Geometry: final body of the model. Coordinates: model frame, mm. Face numbers are marked on the shaded views. A direction names the side the tool comes from. Give positions to 0.01 mm unless a question says otherwise; leave off trailing zeros. Loops run counter-clockwise (first coordinate to the right, second up) from the corner with the lowest first, then second, coordinate; pieces in that order, holes last.
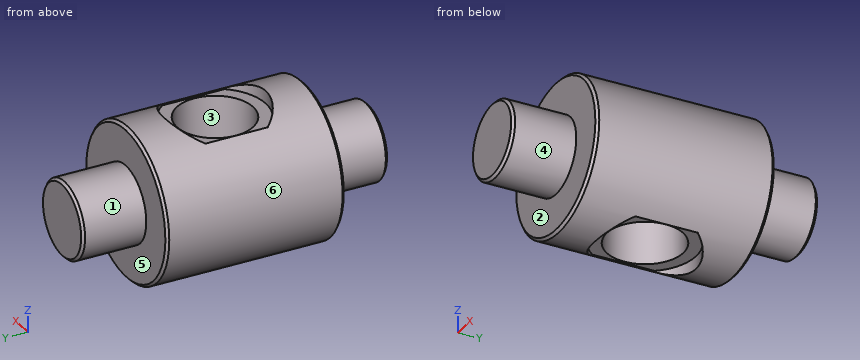
```python
from build123d import *

# Parameters (mm, degrees)
SKETCH1_R           = 1.5
BOSS_EXTRUDE1_DEPTH = 6
SKETCH2_R           = 3
BOSS_EXTRUDE2_DEPTH = 3.5
CUT_EXTRUDE1_DEPTH  = 0.5
SKETCH3_3_R         = 1.5
CUT_EXTRUDE2_DEPTH  = 10.0000001
CHAMFER1_SIZE       = 0.1


with BuildPart() as part:
    # Sketch1 → Boss-Extrude1 (new, symmetric)
    with BuildSketch(Plane(origin=(0, 0, 0), x_dir=(1, 0, 0), z_dir=(0, 1, 0))):
        with Locations(Location((0, 0, 0), (0, 0, 270))):
            Circle(SKETCH1_R)
    extrude(amount=BOSS_EXTRUDE1_DEPTH, both=True)

    # Sketch2 → Boss-Extrude2 (add, symmetric)
    with BuildSketch(Plane(origin=(0, 0, 0), x_dir=(1, 0, 0), z_dir=(0, 1, 0))):
        with Locations(Location((0, 0, 0), (0, 0, 270))):
            Circle(SKETCH2_R)
    extrude(amount=BOSS_EXTRUDE2_DEPTH, both=True)

    # Sketch3 → Cut-Extrude1 (cut)
    with BuildSketch(Plane.XY.offset(3)):
        with BuildLine():
            Line((1.581457004, 1.224334), (1.581457004, -1.224334))
            ThreePointArc((1.581457004, -1.224334), (0, -2), (-1.581457004, -1.224334))
            Line((-1.581457004, -1.224334), (-1.581457004, 1.224334))
            ThreePointArc((-1.581457004, 1.224334), (0, 2), (1.581457004, 1.224334))
        make_face()
    cut_extrude1 = extrude(amount=-CUT_EXTRUDE1_DEPTH, mode=Mode.SUBTRACT)

    # Sketch3_3 → Cut-Extrude2 (cut, through all)
    with BuildSketch(Plane.XY.offset(3)):
        Circle(SKETCH3_3_R)
    extrude(amount=-CUT_EXTRUDE2_DEPTH, mode=Mode.SUBTRACT)

    # Mirror1: Cut-Extrude1 across plane
    add(cut_extrude1.mirror(Plane.XY), mode=Mode.SUBTRACT)

    # Chamfer1
    chamfer1_edges = [part.edges().sort_by_distance(p)[0] for p in [
        (0, -6, -1.5),
        (0, 6, -1.5),
        (0, -3.5, -3),
        (0, 3.5, -3),
    ]]
    chamfer(chamfer1_edges, length=CHAMFER1_SIZE)


solid = part.part
```
Q1. Section query A-A, the plane y = 0. Return loops of the section in (x, z).
Q2. Section query C-C, the plane z = 0. Return loops of the section in (x, y).
Q3. Section query D-D, the plane y = -2.5. Return loops of the section in (x, z), and give its area (3 significant figures).
Q4. Material intervals for probe 1 along Y at (x, z) = (0, 1.1); probe 2 along X at (y, z) = (-5.5, 0); probe 3 along Y at (x, z) = (0.5, -0.25), sorted ascending.
Q5. Mould query, pull axis X, two halves, no side actions, for the marked faces 1, 2 and 3. Classes: +X half, -X half, draft (parallel to the pull), parting line (faces both ways), or undercut.
Q6. Reachability of the marked faces 4, 5 and 6 from +Z, -Z, +X, -X, +Y, -Y: full face, straight path, thin tool, end or side. Return the list, or none.
Q7. Pin query (flat end, axial travel): pin 1 Ø2.5 at (x, y) = (-0.5, -0.5) entering from -Z; pin 2 Ø1.5 at (y, z) = (4, 1) entering from +X; pin 3 Ø1.5 at (y, z) = (-4, 1.5) entering from -X. Return the tip coordinate at first contact, or that it passes through.
Resolved:
1. outline: (-1.58, -2.55) - (-1.58, -2.5) - (-1.5, -2.5) - (-1.5, 2.5) - (-1.58, 2.5) - (-1.58, 2.55) arc R3 ccw to start; (1.5, -2.5) - (1.58, -2.5) - (1.58, -2.55) arc R3 ccw to (1.58, 2.55) - (1.58, 2.5) - (1.5, 2.5) - close
2. outline: (-3, -3.4) - (-2.9, -3.5) - (-1.5, -3.5) - (-1.5, -5.9) - (-1.4, -6) - (1.4, -6) - (1.5, -5.9) - (1.5, -3.5) - (2.9, -3.5) - (3, -3.4) - (3, 3.4) - (2.9, 3.5) - (1.5, 3.5) - (1.5, 5.9) - (1.4, 6) - (-1.4, 6) - (-1.5, 5.9) - (-1.5, 3.5) - (-2.9, 3.5) - (-3, 3.4) - close; hole circle Ø3 at (0, 0)
3. outline: circle Ø6 at (0, 0)
3. area: 28.3 mm2
4. probe 1: y = -6 to -1.5, 1.5 to 6
4. probe 2: x = -1.5 to 1.5
4. probe 3: y = -6 to -1.41, 1.41 to 6
5. face 1: parting line
5. face 2: draft
5. face 3: undercut
6. face 4: -Y
6. face 5: +Y
6. face 6: +Y, -Y
7. pin 1: stops at z = -2.55
7. pin 2: stops at x = 2.95
7. pin 3: stops at x = -2.81
